Build history of the part. All positions in model axes, mm. A direction names the side the tool comes from. Give positions to 0.01 mm unless a question says otherwise; leave off trailing zeros. Loops run counter-clockwise (first coordinate to the right, second up) from the corner with the lowest first, then second, coordinate; pieces in that order, holes last.
1) Band-saw the part on B-B on y = -13.75. List the corners of the cut face in (x, z).
2) 3-axis set-ups, long thin cutter, end or side, ignore diameter. For faces 1 (the flat face through (0, -8, -2.887)), 2 (the flat face through (0, -14, -32.887)), 3 (the flat face through (0, -14, 2.887)): which of +Z, -Z, +X, -X, +Y, -Y reach the whole face in a straight line?
3) Band-saw the part on C-C on x = 7. List the corners of the cut face in (y, z), then the cut area to 3 significant figures.
4) Band-saw the part on D-D on z = 9.5. List the corners of the cut face in (x, y).
5) Two-plate mould, pull along X, no slides. Class faces 4 (the flat face through (27, -21, -12.887)), 5 (the cylindrical face through (9.86, 0.91, -0.04)), 6 (the cylindrical face through (31, -23.51, -0.21)): +X half, -X half, draft (parallel to the pull), parting line (faces both ways), or undercut.
6) Flat gauge pins, fed straight in: P1, Ø10, axis at x = -13.51, y = -27.26, coming from the -Z side; P2, Ø12, axis at x = -13.51, y = -0.24, coming from the +Z side; P3, Ø1.5, axis at y = -10.5, z = -7, coming from the -X side. Where does each tip first touch, or does it go through?
7) Wall check: line 1 (X direction, y = -13.5, z = 9.5); line 2 (Y direction, x = 1, z = 4); line 3 (Z direction, x = 2.5, y = 11). Give the ranges that are in metal, low to high.
8) Band-saw the part on A-A on x = 15.5. List the corners of the cut face in (y, z), then the cut area to 3 significant figures.
```python
from build123d import *

# Parameters (mm, degrees)
SKETCH4_W           = 5.773195876
SKETCH4_H           = 27.5
SKETCH5_R           = 3.827192532
CUT_EXTRUDE1_DEPTH  = 10
SKETCH7_R           = 2.5
BOSS_EXTRUDE1_DEPTH = 30


with BuildPart() as part:
    # Sketch4 → Revolve3 (revolve)
    with BuildSketch(Plane(origin=(0, 0, 0), x_dir=(0, 0, -1), z_dir=(1, 0, 0)), mode=Mode.PRIVATE) as revolve3_sk:
        Polygon((-2.886597938, 13.75), (2.886597938, 13.75), (12.886597938, 13.75), (12.886597938, 18.75), (-12.113402062, 18.75), (-12.113402062, 13.75), align=None)
        Rectangle(SKETCH4_W, SKETCH4_H)
    revolve(revolve3_sk.sketch.rotate(Axis((0, -13.75, 14.432989691), (0, 0, -1)), 90), axis=Axis((0, -13.75, 14.432989691), (0, 0, -1)))

    # Sketch5 → Cut-Extrude1 (cut)
    with BuildSketch(Plane(origin=(0, 0, -2.886597938), x_dir=(-1, 0, 0), z_dir=(0, 0, -1))):
        with Locations((4.945213264, 4.705787154)):
            Circle(SKETCH5_R)
        with Locations(Location((13.51057389, -0.23942611, 0), (0, 0, 180))):
            Circle(SKETCH5_R)
        with Locations((18.455787154, -8.804786736)):
            Circle(SKETCH5_R)
        with Locations(Location((18.455787154, -18.695213264, 0), (0, 0, 180))):
            Circle(SKETCH5_R)
        with Locations((13.51057389, -27.26057389)):
            Circle(SKETCH5_R)
        with Locations(Location((4.945213264, -32.205787154, 0), (0, 0, 180))):
            Circle(SKETCH5_R)
        with Locations((-4.945213264, -32.205787154)):
            Circle(SKETCH5_R)
        with Locations(Location((-13.51057389, -27.26057389, 0), (0, 0, 180))):
            Circle(SKETCH5_R)
        with Locations((-18.455787154, -18.695213264)):
            Circle(SKETCH5_R)
        with Locations(Location((-18.455787154, -8.804786736, 0), (0, 0, 180))):
            Circle(SKETCH5_R)
        with Locations((-13.51057389, -0.23942611)):
            Circle(SKETCH5_R)
        with Locations(Location((-4.945213264, 4.705787154, 0), (0, 0, 180))):
            Circle(SKETCH5_R)
    extrude(amount=-CUT_EXTRUDE1_DEPTH, mode=Mode.SUBTRACT)

    # Sketch7 → Boss-Extrude1 (add)
    with BuildSketch(Plane(origin=(0, 0, -2.886597938), x_dir=(-1, 0, 0), z_dir=(0, 0, -1))):
        with Locations(Location((0, -13.75, 0), (0, 0, 180))):
            Circle(SKETCH7_R)
    extrude(amount=BOSS_EXTRUDE1_DEPTH)


solid = part.part
```
Findings below:
1. outline: (-32.5, -12.89) - (-27.5, -12.89) - (-27.5, -2.89) - (-2.5, -2.89) - (-2.5, -32.89) - (2.5, -32.89) - (2.5, -2.89) - (27.5, -2.89) - (27.5, -12.89) - (32.5, -12.89) - (32.5, 12.11) - (27.5, 12.11) - (27.5, 2.89) - (-27.5, 2.89) - (-27.5, 12.11) - (-32.5, 12.11) - close
2. face 1: -Z
2. face 2: -Z, +X, -X, +Y, -Y
2. face 3: +Z
3. outline: (-45.49, -12.89) - (-40.34, -12.89) - (-40.34, -2.89) - (-35.43, -2.89) - (-35.43, 2.89) - (-40.34, 2.89) - (-40.34, 12.11) - (-45.49, 12.11) - close; (-28.98, -2.89) - (1.48, -2.89) - (1.48, 2.89) - (-28.98, 2.89) - close; (7.93, -2.89) - (12.84, -2.89) - (12.84, -12.89) - (17.99, -12.89) - (17.99, 12.11) - (12.84, 12.11) - (12.84, 2.89) - (7.93, 2.89) - close
3. area: 490 mm2
4. outline: circle Ø65 at (0, -13.75); hole circle Ø55 at (0, -13.75)
5. face 4: draft
5. face 5: undercut
5. face 6: parting line
6. P1: stops at z = -2.89
6. P2: stops at z = 2.89
6. P3: stops at x = -32.4
7. line 1: x = -32.5 to -27.5, 27.5 to 32.5
7. line 2: y = -46.23 to -41.23, 13.73 to 18.73
7. line 3: z = -2.89 to 2.89
8. outline: (-42.32, -12.89) - (-36.47, -12.89) - (-36.47, -2.89) - (-30.53, -2.89) - (-30.53, 2.89) - (-36.47, 2.89) - (-36.47, 12.11) - (-42.32, 12.11) - close; (-23.99, -2.89) - (-21.13, -2.89) - (-21.13, 2.89) - (-23.99, 2.89) - close; (-16.26, -2.89) - (-11.24, -2.89) - (-11.24, 2.89) - (-16.26, 2.89) - close; (-6.37, -2.89) - (-3.51, -2.89) - (-3.51, 2.89) - (-6.37, 2.89) - close; (3.03, -2.89) - (8.97, -2.89) - (8.97, -12.89) - (14.82, -12.89) - (14.82, 12.11) - (8.97, 12.11) - (8.97, 2.89) - (3.03, 2.89) - close
8. area: 423 mm2
